Source: CAD feature listing. Evaluate the final solid. Frame: model axes, mm. Face numbers are marked on the shaded views. A direction names the side the tool comes from. Round coordinates to 2 decimals unless told otherwise and drop trailing zeros. Order: outer loops, then holes, each group sorted by start corner. A loop starts at its lowest first (then second) coordinate and runs counter-clockwise, first axis right, second up. Notation, with made-up numbers: (43.25, -34) - (91.25, -34) arc R13 cw to (91.25, -25) - close; hole circle Ø10 at (1.5, -14). An arc over 180 degrees is marked (long way). Use one line per item in the form item = value. Start each with the question number.
Q1. Ray query, line 1 (X direction, y = 9.5, z = 0); line 2 (X direction, y = 57, z = 0); line 3 (Y direction, x = -14.5, z = -22.5). Return the intervals inside material, ascending. Write a range as [from, to].
Q2. Pin query (flat end, axial travel): pin 1 Ø6 at (x, z) = (5.5, -15.5) entering from -Y; pin 2 Ø2 at (y, z) = (23.5, -14) entering from +X; pin 3 Ø10 at (x, y) = (-16, 8) entering from -Z. Return the tip coordinate at first contact, or that it passes through.
Q3. Set-up query: the marked faces 1 and 2. Return all of +Z, -Z, +X, -X, +Y, -Y with unobstructed straight access to the full face (end or side cutting, diameter ignored); none if empty.
Q4. Cut plane B-B, the plane x = 0. Return the cut outline in (y, z).
Q5. Cut plane C-C, the plane y = 8. Return the cut outline in (x, z), and give its area (3 significant figures).
Q6. Draft query along X for the marked faces 3, 4 and 5. Return one class per face: released by +X, released by -X, zero draft, split by the parting line, or undercut.
Q7. Cut plane A-A, the plane z = 0. Return the cut outline in (x, y).
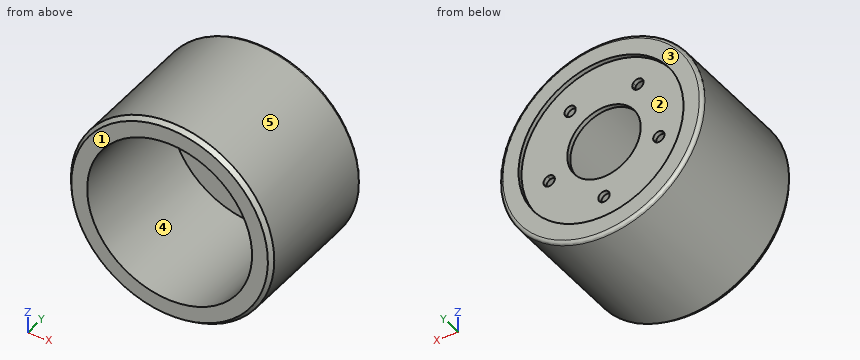
from build123d import *

# Parameters (mm, degrees)
SKETCH3_R           = 45
SKETCH3_R_2         = 36.5
BOSS_EXTRUDE1_DEPTH = 60
FILLET1_R           = 1.5
BOSS_EXTRUDE3_START = 56
SKETCH3_6_R         = 36.5
SKETCH3_6_R_2       = 16.25
BOSS_EXTRUDE3_DEPTH = 2
CHAMFER2_SIZE       = 1.5
CHAMFER2_SIZE2      = 2


with BuildPart() as part:
    # Sketch3 → Boss-Extrude1 (new body)
    with BuildSketch(Plane(origin=(0, 0, 0), x_dir=(1, 0, 0), z_dir=(0, 1, 0))):
        with Locations(Location((0, 0, 0), (0, 0, 270))):
            Circle(SKETCH3_R)
        with Locations(Location((0, 0, 0), (0, 0, 270))):
            Circle(SKETCH3_R_2, mode=Mode.SUBTRACT)
    extrude(amount=BOSS_EXTRUDE1_DEPTH)

    # Fillet1
    fillet1_edges = [part.edges().sort_by_distance(p)[0] for p in [
        (0, 60, -45),
    ]]
    fillet(fillet1_edges, radius=FILLET1_R)

    # Sketch3_6 → Boss-Extrude3 (add)
    # profile 1 of 2: a face of its own
    with BuildSketch(Plane(origin=(0, 0, 0), x_dir=(1, 0, 0), z_dir=(0, 1, 0)).offset(BOSS_EXTRUDE3_START)):
        with Locations(Location((0, 0, 0), (0, 0, 270))):
            Circle(SKETCH3_6_R)
        with BuildLine():
            ThreePointArc((24.926117797, 5.473486235), (25.371095031, 2.75280528), (25.52, 0))
            ThreePointArc((25.52, 0), (23.278681642, -10.45817293), (16.948418414, -19.07934782))
            ThreePointArc((16.948418414, -19.07934782), (17.358281647, -19.815555733), (17.500279639, -20.646113696))
            ThreePointArc((17.500279639, -20.646113696), (15.714342937, -23.041967116), (12.908188753, -22.014746492))
            ThreePointArc((12.908188753, -22.014746492), (0, -25.52), (-12.908188753, -22.014746492))
            ThreePointArc((-12.908188753, -22.014746492), (-16.469742769, -22.668656182), (-16.948418414, -19.07934782))
            ThreePointArc((-16.948418414, -19.07934782), (-24.270962296, -7.886113696), (-24.926117797, 5.473486235))
            ThreePointArc((-24.926117797, 5.473486235), (-26.648603587, 8.658656182), (-23.382887389, 10.223061056))
            ThreePointArc((-23.382887389, 10.223061056), (-15.000279639, 20.646113696), (-2.496999253, 25.397547022))
            ThreePointArc((-2.496999253, 25.397547022), (-0.06124487, 28.019249701), (2.5, 25.52))
            ThreePointArc((2.5, 25.52), (2.499249701, 25.45875513), (2.496999253, 25.397547022))
            ThreePointArc((2.496999253, 25.397547022), (15.000279639, 20.646113696), (23.382887389, 10.223061056))
            ThreePointArc((23.382887389, 10.223061056), (25.690436271, 9.944048009), (26.770962296, 7.886113696))
            ThreePointArc((26.770962296, 7.886113696), (26.256898946, 6.36754344), (24.926117797, 5.473486235))
        make_face(mode=Mode.SUBTRACT)
    # profile 2 of 2: a face of its own
    with BuildSketch(Plane(origin=(0, 0, 0), x_dir=(1, 0, 0), z_dir=(0, 1, 0)).offset(BOSS_EXTRUDE3_START)):
        with BuildLine():
            ThreePointArc((16.948418414, -19.07934782), (23.278681642, -10.45817293), (25.52, 0))
            ThreePointArc((25.52, 0), (25.371095031, 2.75280528), (24.926117797, 5.473486235))
            ThreePointArc((24.926117797, 5.473486235), (21.893321005, 7.113571211), (23.382887389, 10.223061056))
            ThreePointArc((23.382887389, 10.223061056), (15.000279639, 20.646113696), (2.496999253, 25.397547022))
            ThreePointArc((2.496999253, 25.397547022), (0, 23.02), (-2.496999253, 25.397547022))
            ThreePointArc((-2.496999253, 25.397547022), (-15.000279639, 20.646113696), (-23.382887389, 10.223061056))
            ThreePointArc((-23.382887389, 10.223061056), (-22.213027984, 9.305587672), (-21.770962296, 7.886113696))
            ThreePointArc((-21.770962296, 7.886113696), (-22.75239204, 5.900177047), (-24.926117797, 5.473486235))
            ThreePointArc((-24.926117797, 5.473486235), (-24.270962296, -7.886113696), (-16.948418414, -19.07934782))
            ThreePointArc((-16.948418414, -19.07934782), (-14.169721675, -18.288111688), (-12.500279639, -20.646113696))
            ThreePointArc((-12.500279639, -20.646113696), (-12.604426219, -21.360176995), (-12.908188753, -22.014746492))
            ThreePointArc((-12.908188753, -22.014746492), (0, -25.52), (12.908188753, -22.014746492))
            ThreePointArc((12.908188753, -22.014746492), (13.530816508, -18.623571211), (16.948418414, -19.07934782))
        make_face()
        with Locations(Location((0, 0, 0), (0, 0, 270))):
            Circle(SKETCH3_6_R_2, mode=Mode.SUBTRACT)
    extrude(amount=BOSS_EXTRUDE3_DEPTH)

    # Chamfer2
    chamfer2_edges = [part.edges().sort_by_distance(p)[0] for p in [
        (0, 0, -45),
    ]]
    chamfer2_side = [part.faces().sort_by_distance(p)[0] for p in [
        (0, 0, -43.727207794),
    ]]
    chamfer(chamfer2_edges, length=CHAMFER2_SIZE, length2=CHAMFER2_SIZE2, reference=chamfer2_side[0])


solid = part.part
Completed:
q1.line_1 = [-45, -36.5], [36.5, 45]
q1.line_2 = [-45, -16.25], [16.25, 45]
q1.line_3 = [56, 58]
q2.pin_1 = 56
q2.pin_2 = 43.08
q2.pin_3 = -43.63
q3.face_1 = +Z, -Z, +X, -X, -Y
q3.face_2 = +Y
q4.outline = (0, -43.5) - (2, -45) - (58.5, -45) arc R1.5 ccw to (60, -43.5) - (60, -36.5) - (58, -36.5) - (58, -28.02) - (56, -28.02) - (56, -36.5) - (0, -36.5) - close; (0, 36.5) - (56, 36.5) - (56, 16.25) - (58, 16.25) - (58, 36.5) - (60, 36.5) - (60, 43.5) arc R1.5 ccw to (58.5, 45) - (2, 45) - (0, 43.5) - close; (56, -23.02) - (58, -23.02) - (58, -16.25) - (56, -16.25) - close
q5.outline = circle Ø90 at (0, 0); hole circle Ø73 at (0, 0)
q5.area = 2,180 mm2
q6.face_3 = zero draft
q6.face_4 = undercut
q6.face_5 = split by the parting line
q7.outline = (-45, 2) - (-43.5, 0) - (-36.5, 0) - (-36.5, 56) - (-16.25, 56) - (-16.25, 58) - (-36.5, 58) - (-36.5, 60) - (-43.5, 60) arc R1.5 ccw to (-45, 58.5) - close; (16.25, 56) - (36.5, 56) - (36.5, 0) - (43.5, 0) - (45, 2) - (45, 58.5) arc R1.5 ccw to (43.5, 60) - (36.5, 60) - (36.5, 58) - (16.25, 58) - close
